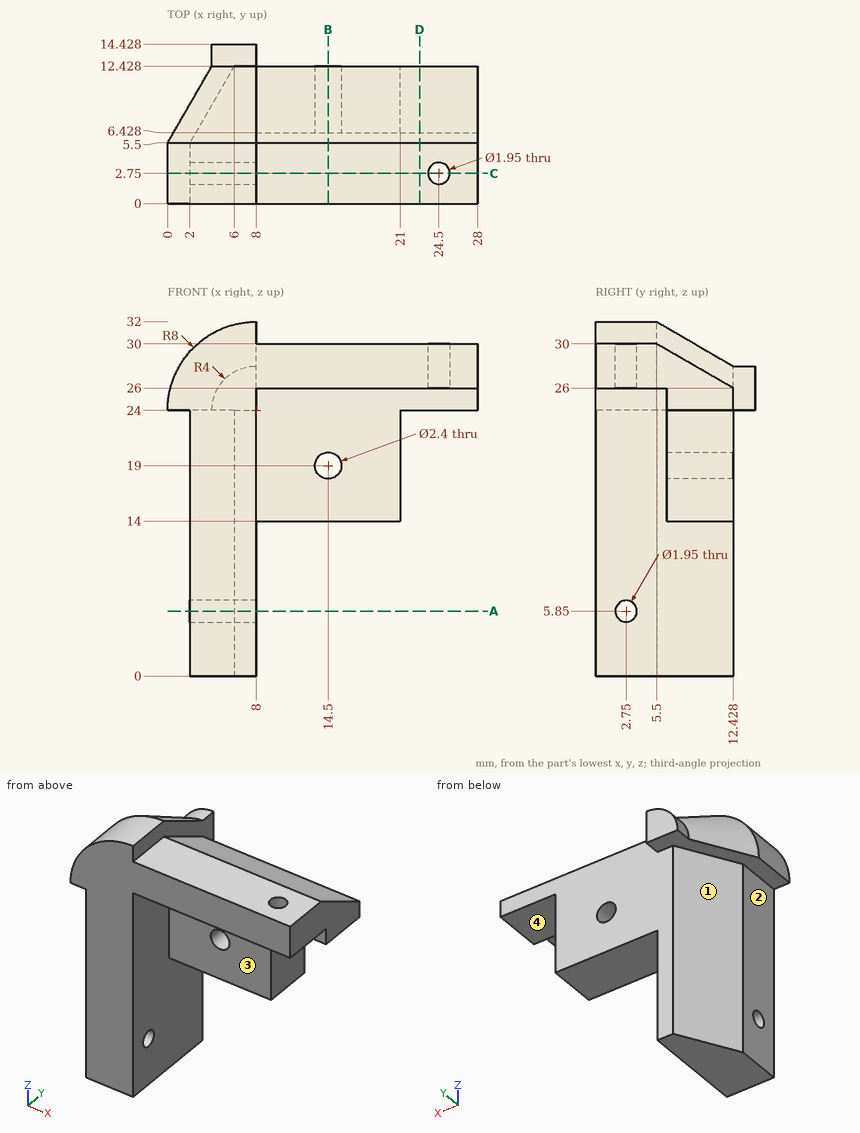
Drawing for the job (mm, zero at the part's lowest x, y, z). A direction names the side the tool comes from. Coordinates: 2 decimals unless noted, no trailing zeros. Write each loop counter-clockwise with the first axis right and the second up, starting at its lowest first coordinate (ties: lowest second). Pieces come first, ordered by that corner, then holes. Notation, with made-up numbers: (65, 40.5) -> (91, 40.5) arc R32 cw to (91, 72.5) -> close; hole circle Ø5 at (37, -9.5). An arc over 180 degrees is marked (long way). One line per item, written item: value. Start each with the question number.
1) Probe probe 1 along Y at (x, z) = (6.15, 5.85) (1 decimal); probe 2 along Z at (x, y) = (13.75, 9.5); probe 3 along Z at (x, y) = (15, 4.75). List the from-to ranges inside material, lowest first.
2) Slice it at B-B on x = 14.5. Write the cut outline in (y, z).
3) Slice it at D-D on x = 22.75. Write the cut outline in (y, z).
4) Slice it at C-C on y = 2.75. Write the cut outline in (x, z) (3 decimals).
5) Which spindle directions (+Z, -Z, +X, -X, +Y, -Y) get a long thin tool onto all of the face, cutting with end or side? Do the marked faces 1, 2, 3 and 4. Say none if no direction does.
6) Slice it at A-A on z = 5.85. Write the cut outline in (x, y) (1 decimal).
7) Flat gauge pins, fed straight in: pin 1 Ø9.5 at (x, z) = (21.5, 18.5) entering from -Y; pin 2 Ø3.5 at (y, z) = (4, 19) entering from +X; pin 3 Ø2 at (y, z) = (5.5, 7.5) entering from -X; pin 4 Ø4 at (y, z) = (6.5, 29.5) entering from +X. Where does each tip first touch, or does it go through?
Answers follow:
1. probe 1: 0 to 1.8, 3.7 to 12.4
1. probe 2: 14 to 18.06, 19.94 to 27.69
1. probe 3: 26 to 30
2. outline: (0, 26) -> (6.43, 26) -> (6.43, 20.2) -> (12.43, 20.2) -> (12.43, 26) -> (5.5, 30) -> (0, 30) -> close; (6.43, 14) -> (12.43, 14) -> (12.43, 17.8) -> (6.43, 17.8) -> close
3. outline: (0, 26) -> (6.43, 26) -> (6.43, 24) -> (12.43, 24) -> (12.43, 26) -> (5.5, 30) -> (0, 30) -> close
4. outline: (0, 24) -> (2, 24) -> (2, 6.825) -> (8, 6.825) -> (8, 26) -> (23.525, 26) -> (23.525, 30) -> (8, 30) -> (8, 32) arc R8 ccw to start; (2, 0) -> (8, 0) -> (8, 4.875) -> (2, 4.875) -> close; (25.475, 26) -> (28, 26) -> (28, 30) -> (25.475, 30) -> close
5. face 1: -Z, -X, +Y
5. face 2: -Z, -X, +Y, -Y
5. face 3: -Z, +X, -Y
5. face 4: -Z, +X, +Y, -Y
6. outline: (2, 0) -> (8, 0) -> (8, 1.8) -> (2, 1.8) -> close; (2, 3.7) -> (8, 3.7) -> (8, 12.4) -> (6, 12.4) -> (2, 5.5) -> close
7. pin 1: y = 6.43
7. pin 2: x = 8
7. pin 3: x = 2
7. pin 4: x = 28
